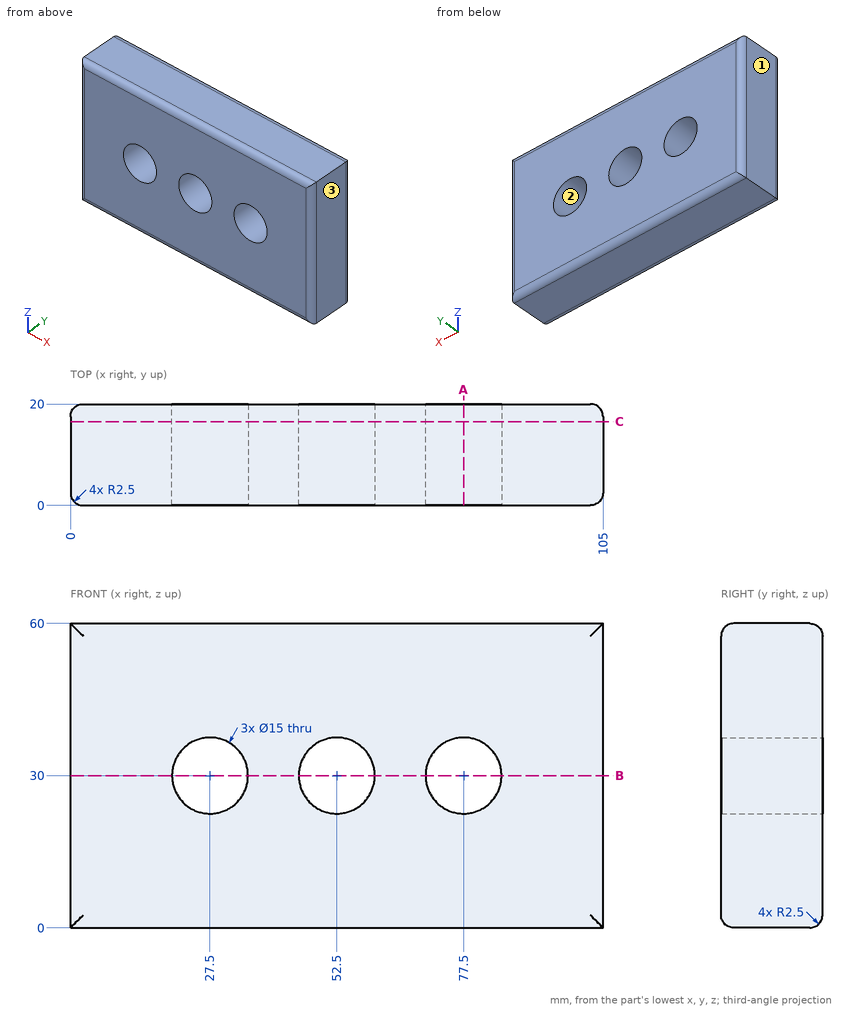
Answer from the drawing. Dimensions are ordinates in mm from the lowest x, y and z of the part. Round coordinates to 2 decimals unless told otherwise and drop trailing zeros. Write each loop counter-clockwise with the first axis right and the second up, starting at its lowest first coordinate (ties: lowest second). Pieces come first, ordered by that corner, then holes. Notation, with made-up numbers: M 47.25,80.5 L 78.25,80.5 A5 cw 78.25,85.5 Z; hole C 70,23 d3. An arc over 180 degrees is marked long. Write each question's results on one line, items separated by ' | '. Start each with the question number.
Item 1: Flat-ended cylindrical pins translate along their axes: pin 1 Ø1.5 at (y, z) = (8, 43) entering from -X; pin 2 Ø13.5 at (x, z) = (27.5, 30) entering from +Y. Find the tip coordinate at first contact, or state that the pin passes through.
Item 2: A cutting plane is placed at A-A on x = 77.5. Write down the section's boundary in (y, z).
Item 3: A cutting plane is placed at B-B on z = 30. Write down the section's boundary in (x, y), and give its area (3 significant figures).
Item 4: For a pull along X with two mould halves and no side action, classify the marked faces 1, 2 and 3 as pulls with the +X half, pulls with the -X half, needs draft (parallel to the pull), parting line crosses it, or undercut.
Item 5: Straight lines are drawn through the part: L1, parallel to Z at x = 27.5, y = 12.25; L2, parallel to X at y = 2.25, z = 39; L3, parallel to Z at x = 79.5, y = 15. For each, find the intervals that lie inside material, in ascending order. Write a range as [from, to].
Item 6: A cutting plane is placed at C-C on y = 16.5. Write down the section's boundary in (x, z).
Check sheet entries:
1) pin 1: x = 0 | pin 2: through
2) outline: M 0,2.5 A2.5 ccw 2.5,0 L 17.5,0 A2.5 ccw 20,2.5 L 20,22.5 L 0,22.5 Z; M 0,37.5 L 20,37.5 L 20,57.5 A2.5 ccw 17.5,60 L 2.5,60 A2.5 ccw 0,57.5 Z
3) outline: M 0,2.5 A2.5 ccw 2.5,0 L 20,0 L 20,20 L 2.5,20 A2.5 ccw 0,17.5 Z; M 35,0 L 45,0 L 45,20 L 35,20 Z; M 60,0 L 70,0 L 70,20 L 60,20 Z; M 85,0 L 102.5,0 A2.5 ccw 105,2.5 L 105,17.5 A2.5 ccw 102.5,20 L 85,20 Z | area: 1,190 mm²
4) face 1: pulls with the -X half | face 2: undercut | face 3: pulls with the +X half
5) L1: [0, 22.5], [37.5, 60] | L2: [0.01, 104.99] | L3: [0, 22.77], [37.23, 60]
6) outline: M 0,0 L 105,0 L 105,60 L 0,60 Z; hole C 27.5,30 d15; hole C 52.5,30 d15; hole C 77.5,30 d15
